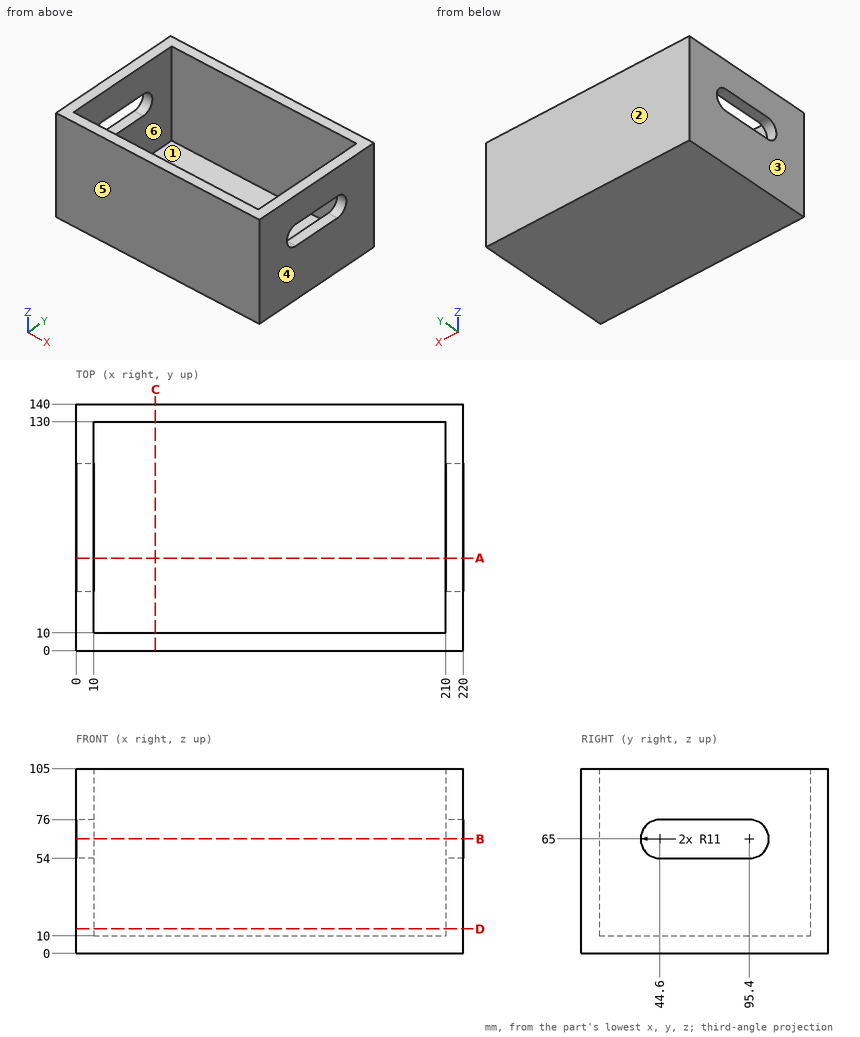
Here's the drawing with two shaded views (mm, measured from the low corner). I have some questions. A direction names the side the tool comes from. Coordinates: 2 decimals unless noted, no trailing zeros. Write each loop counter-clockwise with the first axis right and the second up, starting at its lowest first coordinate (ties: lowest second). Pieces come first, ordered by that corner, then holes.
Item 1: If we mould it in two halves opening along X, with no side actions, what happens to the marked faces 3, 4, 5 and 6? For each: +X half, -X half, draft (parallel to the pull), parting line (faces both ways), or undercut.
Item 2: I want a section at B-B on z = 65. Write out the boundary of the cut face in (x, y), and give its area (3 significant figures).
Item 3: On a 3-axis mill with a long thin cutter (end or side, diameter ignored), from which of +Z, -Z, +X, -X, +Y, -Y can I reach the whole of each face in a straight line? I mean the marked faces 1 and 2. Say none if no direction works.
Item 4: If I drill on line 1 (Y direction, x = 62, z = 71.5); line 2 (X direction, y = 125, z = 24.5); line 3 (Z direction, x = 54, y = 64.5), over which ranges is the centre line in solid material (lowest first)?
Item 5: Will this pin go through, and if not, where does the flat tip stop? pin 1 (12 mm diameter, centred on x = 116, y = 48.5, fed in from +Z).
Item 6: I want a section at C-C on x = 45. Write out the boundary of the cut face in (y, z).
Item 7: I want a section at A-A on y = 52.5. Write out the boundary of the cut face in (x, z), and give its area (3 significant figures).
Item 8: I want a section at D-D on z = 14. Write out the boundary of the cut face in (x, y), and give its area (3 significant figures).
Findings below:
1. face 3: -X half
1. face 4: +X half
1. face 5: draft
1. face 6: undercut
2. outline: (0, 0) - (220, 0) - (220, 33.6) - (210, 33.6) - (210, 10) - (10, 10) - (10, 33.6) - (0, 33.6) - close; (0, 106.4) - (10, 106.4) - (10, 130) - (210, 130) - (210, 106.4) - (220, 106.4) - (220, 140) - (0, 140) - close
2. area: 5,340 mm2
3. face 1: +Z
3. face 2: +Z, -Z, +X, -X, +Y
4. line 1: y = 0 to 10, 130 to 140
4. line 2: x = 0 to 10, 210 to 220
4. line 3: z = 0 to 10
5. pin 1: stops at z = 10
6. outline: (0, 0) - (140, 0) - (140, 105) - (130, 105) - (130, 10) - (10, 10) - (10, 105) - (0, 105) - close
7. outline: (0, 0) - (220, 0) - (220, 54) - (210, 54) - (210, 10) - (10, 10) - (10, 54) - (0, 54) - close; (0, 76) - (10, 76) - (10, 105) - (0, 105) - close; (210, 76) - (220, 76) - (220, 105) - (210, 105) - close
7. area: 3,660 mm2
8. outline: (0, 0) - (220, 0) - (220, 140) - (0, 140) - close; hole (10, 10) - (210, 10) - (210, 130) - (10, 130) - close
8. area: 6,800 mm2
